Autodesk Inventor part; units mm, degrees
ref_plane "YZ Plane" through (0, 0, 0) normal (1, 0, 0) x (0, 1, 0)
ref_plane "XZ Plane" through (0, 0, 0) normal (0, 1, 0) x (-1, 0, 0)
ref_plane "XY Plane" through (0, 0, 0) normal (0, 0, 1) x (1, 0, 0)
sketch "Sketch1" plane through (0, 0, 0) normal (1, 0, 0) x (0, 1, 0)
  line L0 (0, 0) -> (147, 0)
  line L1 (147, 0) -> (147, 110)
  line L2 (147, 110) -> (0, 110)
  line L3 (0, 110) -> (0, 0)
  circle A0 centre (124.75, 106.25) radius 1
  circle A1 centre (124.75, 3.75) radius 1
  circle A2 centre (22.25, 3.75) radius 1
  circle A3 centre (22.25, 106.25) radius 1
  dimension "d0" = 102.5
  dimension "d1" = 102.5
  dimension "d2" = 2
  dimension "d3" = 110
  dimension "d4" = 147
  dimension "d5" = 22.25
  dimension "d6" = 22.25
  dimension "d7" = 3.75
  dimension "d8" = 3.75
extrude "Extrusion1" add sketch "Sketch1" along normal blind 2
sketch "Sketch5" plane through (2, 0, 0) normal (1, 0, 0) x (0, 0, -1)
  line L0 (0, 0) -> (0, 147)
  line L1 (-110, 147) -> (-110, 0)
  circle A0 centre (-13.8284, 13.0004) radius 1.5
  circle A1 centre (-96.1716, 13.0004) radius 1.5
  circle A2 centre (-89, 136.172) radius 1.5
  circle A3 centre (-96.1716, 105.0004) radius 1.5
  circle A4 centre (-21, 136.172) radius 1.5
  line L2 (-110, 0) -> (0, 0)
  line L3 (0, 147) -> (-110, 147)
  dimension "d94" = 3
  dimension "d116" = 21
  dimension "d117" = 68
  dimension "d118" = 82.3431
  dimension "d119" = 123.1716
  dimension "d120" = 7.1716
  dimension "d121" = 92
  dimension "d122" = 10.828
extrude "Extrusion4" cut sketch "Sketch5" against normal through all contours A0 | A1 | A2 | A3 | A4
sketch "Sketch7" plane through (0, 0, 0) normal (-1, 0, 0) x (0, 0, 1)
  line L0 (21, 59.172) -> (49, 59.172)
  line L1 (49, 59.172) -> (49, 28.172)
  line L2 (49, 28.172) -> (21, 28.172)
  line L3 (21, 28.172) -> (21, 59.172)
  line L4 (71, 27.672) -> (79, 27.672)
  line L5 (79, 27.672) -> (79, 24.672)
  line L6 (79, 24.672) -> (71, 24.672)
  line L7 (71, 24.672) -> (71, 27.672)
  line L8 (66, 66.672) -> (84, 66.672)
  line L9 (84, 66.672) -> (84, 57.672)
  line L10 (84, 57.672) -> (66, 57.672)
  line L11 (66, 57.672) -> (66, 66.672)
  line L12 (25, 81.172) -> (45, 81.172)
  line L13 (45, 81.172) -> (45, 69.172)
  line L14 (45, 69.172) -> (25, 69.172)
  line L15 (25, 69.172) -> (25, 81.172)
  circle A0 centre (75, 19.672) radius 1.5
  circle A1 centre (62.5, 62.172) radius 1
  circle A2 centre (87.5, 62.172) radius 1
  line L16 (21, 131.172) -> (89, 131.172)
  line L17 (21, 128.172) -> (89, 128.172)
  line L18 (21, 125.172) -> (89, 125.172)
  line L19 (21, 122.172) -> (89, 122.172)
  line L20 (21, 119.172) -> (89, 119.172)
  line L21 (21, 131.172) -> (21, 89.172)
  line L22 (89, 131.172) -> (89, 89.172)
  line L23 (21, 116.172) -> (89, 116.172)
  line L24 (21, 113.172) -> (89, 113.172)
  line L25 (21, 110.172) -> (89, 110.172)
  line L26 (21, 107.172) -> (89, 107.172)
  line L27 (21, 104.172) -> (89, 104.172)
  line L28 (21, 89.172) -> (89, 89.172)
  circle A3 centre (21, 136.172) radius 1.5 construction
  circle A4 centre (21, 136.172) radius 1.5
  circle A5 centre (89, 136.172) radius 1.5 construction
  circle A6 centre (89, 136.172) radius 1.5
  line L29 (110, 147) -> (110, 0)
  line L30 (0, 0) -> (0, 147)
  line L31 (21, 101.172) -> (89, 101.172)
  line L32 (89, 98.172) -> (21, 98.172)
  line L33 (21, 95.172) -> (89, 95.172)
  line L34 (21, 92.172) -> (89, 92.172)
  line L35 (66, 79.672) -> (84, 79.672)
  line L36 (84, 79.672) -> (84, 70.672)
  line L37 (84, 70.672) -> (66, 70.672)
  line L38 (66, 70.672) -> (66, 79.672)
  circle A7 centre (62.5, 75.172) radius 1
  circle A8 centre (87.5, 75.172) radius 1
  line L39 (66, 53.672) -> (84, 53.672)
  line L40 (84, 53.672) -> (84, 44.672)
  line L41 (84, 44.672) -> (66, 44.672)
  line L42 (66, 44.672) -> (66, 53.672)
  circle A9 centre (62.5, 49.172) radius 1
  circle A10 centre (87.5, 49.172) radius 1
  line L43 (66, 40.672) -> (84, 40.672)
  line L44 (84, 40.672) -> (84, 31.672)
  line L45 (84, 31.672) -> (66, 31.672)
  line L46 (66, 31.672) -> (66, 40.672)
  circle A11 centre (62.5, 36.172) radius 1
  circle A12 centre (87.5, 36.172) radius 1
  point P0 (35, 69.172)
  point P1 (35, 59.172)
  point P2 (75, 57.672)
  point P3 (75, 27.672)
  point P4 (75, 24.672)
  point P5 (66, 62.172)
  point P6 (84, 62.172)
  point P7 (66, 75.172)
  point P8 (45, 75.172)
  point P9 (66, 49.172)
  point P10 (84, 36.172)
  point P11 (66, 36.172)
  dimension "d105" = 8
  dimension "d106" = 3
  dimension "d107" = 18
  dimension "d108" = 9
  dimension "d109" = 28
  dimension "d110" = 31
  dimension "d111" = 20
  dimension "d112" = 12
  dimension "d123" = 3
  dimension "d124" = 5
  dimension "d125" = 25
  dimension "d126" = 12.5
  dimension "d127" = 2
  dimension "d129" = 3
  dimension "d130" = 3
  dimension "d131" = 3
  dimension "d133" = 3
  dimension "d134" = 3
  dimension "d135" = 3
  dimension "d136" = 3
  dimension "d137" = 3
  dimension "d138" = 3
  dimension "d140" = 5
  dimension "d141" = 40
  dimension "d142" = 35
  dimension "d143" = 35
  dimension "d144" = 10
  dimension "d150" = 3
  dimension "d151" = 3
  dimension "d152" = 3
  dimension "d154" = 3
  dimension "d155" = 3
  dimension "d156" = 8
  dimension "d158" = 4
  dimension "d159" = 4
  dimension "d161" = 4
  dimension "d162" = 4
extrude "Extrusion5" cut sketch "Sketch7" against normal through all contours L0 L1 L2 L3 | L4 L5 L6 L7 | L8 L9 L10 L11 | L12 L13 L14 L15 | A0 | A1 | A2 | L16 L22 L17 L21 | L18 L22 L19 L21 | L20 L22 L23 L21 | L24 L22 L25 L21 | L26 L22 L27 L21 | L31 L22 L32 L21 | L33 L22 L34 L21 | L35 L36 L37 L38 | A7 | A8 | L39 L40 L41 L42 | A9 | A10 | L43 L44 L45 L46 | A11 | A12
equation "\"d1\" = d0"
equation "\"d5\" = d6"
equation "\"d7\" = d8"
properties part number "front plate"
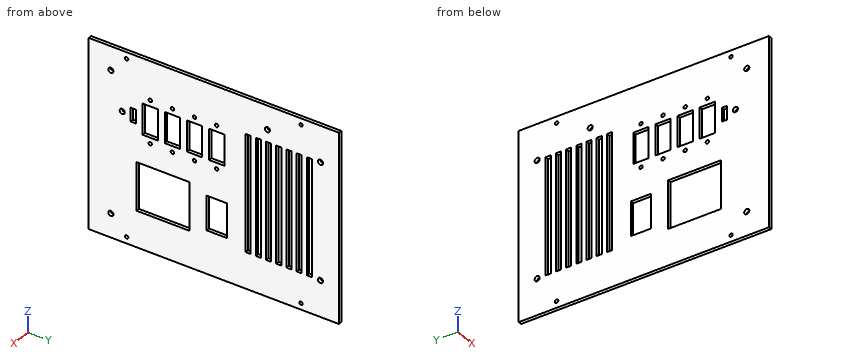
Can you work these out from the model? Positions are in its coordinate system, mm. Coordinates: 2 decimals unless noted, no trailing zeros. Order: outer loops, then holes, each group sorted by start corner. A loop starts at its lowest first (then second) coordinate and runs counter-clockwise, first axis right, second up.
1. If we section it at A-A (y = 72.5): Please give me the cut outline in (x, z), then the cut area to 3 significant figures.
2. I need wall thicknesses on line 1 (Y direction, x = 0.4, z = 106.25); line 2 (Z direction, x = 0.5, y = 62); line 3 (Z direction, x = 1.5, y = 38). Which ranges of each line are inside material? Lowest first, please.
3. If we section it at B-B (z = 58.5): Give the number of separate pieces and of enclosed holes in the cut face, then the cut area to 3 significant figures.
4. I'm going to push flat-ended pins straight in: pin 1 (2 mm diameter, centred on y = 119, z = 92.5, fed in from -X); pin 2 (1.2 mm diameter, centred on y = 49.172, z = 87.5, fed in from -X). Where does each tip first touch, or does it pass through?
Entries:
1. outline: (0, 0) - (2, 0) - (2, 25) - (0, 25) - close; (0, 45) - (2, 45) - (2, 66) - (0, 66) - close; (0, 84) - (2, 84) - (2, 110) - (0, 110) - close
1. area: 144 mm2
2. line 1: y = 0 to 21.25, 23.25 to 123.75, 125.75 to 147
2. line 2: z = 0 to 61.51, 63.49 to 66, 84 to 86.51, 88.49 to 110
2. line 3: z = 0 to 21, 49 to 66, 84 to 110
3. separate pieces: 8
3. enclosed holes: 0
3. area: 252 mm2
4. pin 1: stops at x = 0
4. pin 2: passes through
